```python
from build123d import *

# Parameters (mm, degrees)
F0_W      = 32
F0_H      = 23
F1_DEPTH  = 19
F2_R      = 5
F3_R      = 5
F4_W      = 3
F4_H      = 5
F5_DEPTH  = 5
F7_DEPTH  = 28
F8_R      = 2.5
F9_DEPTH  = 9
F10_R     = 2.5
F11_DEPTH = 9


with BuildPart() as f1:
    # F0 (on Front) → F1 (new body)
    with BuildSketch(Plane.XZ):
        with Locations((16, 11.5)):
            Rectangle(F0_W, F0_H)
    extrude(amount=-F1_DEPTH)

    # F2
    f2_edges = [f1.edges().sort_by_distance(p)[0] for p in [
        (0, 9.5, 23),
    ]]
    fillet(f2_edges, radius=F2_R)

    # F3
    f3_edges = [f1.edges().sort_by_distance(p)[0] for p in [
        (0, 9.5, 0),
    ]]
    fillet(f3_edges, radius=F3_R)

    # F4 (on face) → F5 (join)
    with BuildSketch(Plane(origin=(0, 0, 0), x_dir=(0, -1, 0), z_dir=(-1, 0, 0))):
        with Locations((-9.5, 11.5)):
            Rectangle(F4_W, F4_H)
    extrude(amount=F5_DEPTH)

    # F6 (on face) → F7 (join)
    with BuildSketch(Plane.YZ.offset(32)):
        with BuildLine():
            Line((19, 5.019259), (19, 17.980741))
            ThreePointArc((19, 17.980741), (14.872219, 21.668051), (9.5, 23))
            ThreePointArc((9.5, 23), (4.127781, 21.668051), (0, 17.980741))
            Line((0, 17.980741), (0, 5.019259))
            ThreePointArc((0, 5.019259), (4.127781, 1.331949), (9.5, 0))
            ThreePointArc((9.5, 0), (14.872219, 1.331949), (19, 5.019259))
        make_face()
        with BuildLine():
            ThreePointArc((19, 5.019259), (20.48863, 8.108835), (21, 11.5))
            ThreePointArc((21, 11.5), (20.48863, 14.891165), (19, 17.980741))
            Line((19, 17.980741), (19, 5.019259))
        make_face()
        with BuildLine():
            Line((0, 5.019259), (0, 17.980741))
            ThreePointArc((0, 17.980741), (-2, 11.5), (0, 5.019259))
        make_face()
    extrude(amount=F7_DEPTH)

    # F8 (on face) → F9 (join)
    with BuildSketch(Plane.XZ):
        with Locations((11, 11.5)):
            Circle(F8_R)
    extrude(amount=F9_DEPTH)

    # F10 (on face) → F11 (join)
    with BuildSketch(Plane(origin=(0, 19, 0), x_dir=(-1, 0, 0), z_dir=(0, 1, 0))):
        with Locations((-11, 11.5)):
            Circle(F10_R)
    extrude(amount=F11_DEPTH)


solid = f1.part
```
Input: part model. Units: mm. Frame: model coordinates. A direction names the side the tool comes from. Give positions to 0.01 mm unless a question says otherwise; leave off trailing zeros. Loops run counter-clockwise (first coordinate to the right, second up) from the corner with the lowest first, then second, coordinate; pieces in that order, holes last.
1) Section query A-A on x = 38.5. Return the cut outline in (y, z).
A:
outline: (0, 5.02) arc R11.5 ccw to (9.5, 0) arc R11.5 ccw to (19, 5.02) arc R11.5 ccw to (21, 11.5) arc R11.5 ccw to (19, 17.98) arc R11.5 ccw to (9.5, 23) arc R11.5 ccw to (0, 17.98) arc R11.5 ccw to start
2) Section query C-C on z = 1.75. Return the cut outline in (x, y).
A:
outline: (1.2, 0) - (32, 0) - (32, 3.4) - (60, 3.4) - (60, 15.6) - (32, 15.6) - (32, 19) - (1.2, 19) - close
3) Section query B-B on y = 3. Return the cut outline in (x, z).
A:
outline: (0, 5) arc R5 ccw to (5, 0) - (32, 0) - (32, 2.01) - (60, 2.01) - (60, 20.99) - (32, 20.99) - (32, 23) - (5, 23) arc R5 ccw to (0, 18) - close
4) Contact query for flat-ended pins moving along their axis: pin 1 (5.5 mm diameter, centred on x = -3.5, z = 12, fed in from -Y); pin 2 (1.5 mm diameter, centred on x = 48.5, z = 19.5, fed in from +Y); pin 3 (4 mm diameter, centred on x = -1.5, z = 12.5, fed in from +Y). Output: stop coordinate, or through.
A:
pin 1: stops at y = 8
pin 2: stops at y = 18.43
pin 3: stops at y = 19
5) Section query D-D on x = 11. Return the cut outline in (y, z).
A:
outline: (-9, 9) - (0, 9) - (0, 0) - (19, 0) - (19, 9) - (28, 9) - (28, 14) - (19, 14) - (19, 23) - (0, 23) - (0, 14) - (-9, 14) - close
6) Line query: L1, parallel to Y at x = 4.5, z = 14.75; L2, parallel to X at y = 15, z = 17.75; L3, parallel to Z at x = 56, y = 20. Output: solid intervals per line, ascending.
A:
L1: y = 0 to 19
L2: x = 0 to 60
L3: z = 6.81 to 16.19
7) Reachability of faces 1 (the flat face through (32, -1, 12)), 2 (the cylindrical face through (11.54, 23.44, 9.06)), 3 (the flat face through (32, 2, 22)), 4 (the flat face through (32, 2, 2)) from +Z, -Z, +X, -X, +Y, -Y: full face, straight path, thin tool, end or side. Return the list, or none.
A:
face 1: +Z, -Z, -Y
face 2: +Y
face 3: +Z, +X, -Y
face 4: -Z, +X, -Y
8) Mould query, pull axis X, two halves, no side actions, for faces 5 (the flat face through (11, 28, 12)), 6 (the flat face through (32, 20, 12)), 7 (the flat face through (60, 9, 12)). Classes: released by +X, released by -X, zero draft, split by the parting line, or undercut.
A:
face 5: zero draft
face 6: undercut
face 7: released by +X
